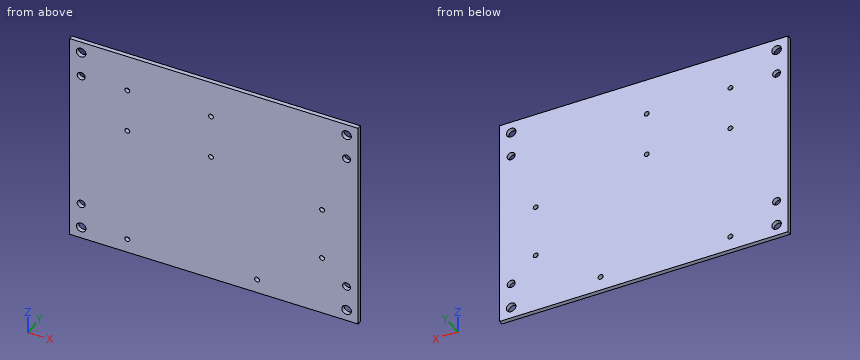
```python
from build123d import *

# Parameters (mm, degrees)
SKETCH1_W           = 200
SKETCH1_H           = 150
BOSS_EXTRUDE1_DEPTH = 3
SKETCH2_R           = 3.3
SKETCH2_R_2         = 1.7
SKETCH2_R_3         = 2.75
SKETCH2_R_4         = 1.75
CUT_EXTRUDE1_DEPTH  = 3


with BuildPart() as part:
    # Sketch1 → Boss-Extrude1 (new body)
    with BuildSketch(Plane(origin=(0, 0, 0), x_dir=(1, 0, 0), z_dir=(0, 1, 0))):
        with Locations((100, 75)):
            Rectangle(SKETCH1_W, SKETCH1_H)
    extrude(amount=BOSS_EXTRUDE1_DEPTH)

    # Sketch2 → Cut-Extrude1 (cut)
    with BuildSketch(Plane(origin=(0, 3, 0), x_dir=(1, 0, 0), z_dir=(0, 1, 0))):
        with Locations(Location((8, 142, 0), (0, 0, 270))):
            Circle(SKETCH2_R)
        with Locations(Location((8, 8, 0), (0, 0, 90))):
            Circle(SKETCH2_R)
        with Locations(Location((192, 8, 0), (0, 0, 270))):
            Circle(SKETCH2_R)
        with Locations(Location((192, 142, 0), (0, 0, 90))):
            Circle(SKETCH2_R)
        with Locations(Location((40, 57, 0), (0, 0, 270))):
            Circle(SKETCH2_R_2)
        with Locations(Location((98, 57, 0), (0, 0, 270))):
            Circle(SKETCH2_R_2)
        with Locations(Location((98, 26, 0), (0, 0, 270))):
            Circle(SKETCH2_R_2)
        with Locations(Location((40, 26, 0), (0, 0, 270))):
            Circle(SKETCH2_R_2)
        with Locations(Location((8, 124, 0), (0, 0, 270))):
            Circle(SKETCH2_R_3)
        with Locations(Location((8, 26, 0), (0, 0, 90))):
            Circle(SKETCH2_R_3)
        with Locations(Location((192, 26, 0), (0, 0, 270))):
            Circle(SKETCH2_R_3)
        with Locations(Location((192, 124, 0), (0, 0, 90))):
            Circle(SKETCH2_R_3)
        with Locations(Location((175, 108, 0), (0, 0, 270))):
            Circle(SKETCH2_R_2)
        with Locations(Location((175, 71.07, 0), (0, 0, 270))):
            Circle(SKETCH2_R_2)
        with Locations(Location((40, 140, 0), (0, 0, 270))):
            Circle(SKETCH2_R_4)
        with Locations(Location((130, 140, 0), (0, 0, 270))):
            Circle(SKETCH2_R_4)
    extrude(amount=-CUT_EXTRUDE1_DEPTH, mode=Mode.SUBTRACT)


solid = part.part
```
Here's how the part is built. I have some questions about the finished solid (model axes, mm). Round coordinates to 2 decimals unless told otherwise and drop trailing zeros. Write each loop counter-clockwise with the first axis right and the second up, starting at its lowest first coordinate (ties: lowest second). Pieces come first, ordered by that corner, then holes.
Q1. If we section it at A-A on z = -124: Write out the boundary of the cut face in (x, y).
Q2. Please list where these lines run through material, in increasing order: probe 1 along X at (y, z) = (1.5, -57); probe 2 along X at (y, z) = (1.4, -124); probe 3 along X at (y, z) = (2.2, -26).
Q3. If we section it at B-B on x = 192: Write out the boundary of the cut face in (y, z).
Q4. Will this pin go through, and if not, where does the flat tip stop? P1, Ø3, axis at x = 130, z = -140, coming from the -Y side.
Answer below:
1. outline: (0, 0) - (5.25, 0) - (5.25, 3) - (0, 3) - close; (10.75, 0) - (189.25, 0) - (189.25, 3) - (10.75, 3) - close; (194.75, 0) - (200, 0) - (200, 3) - (194.75, 3) - close
2. probe 1: x = 0 to 38.3, 41.7 to 96.3, 99.7 to 200
2. probe 2: x = 0 to 5.25, 10.75 to 189.25, 194.75 to 200
2. probe 3: x = 0 to 5.25, 10.75 to 38.3, 41.7 to 96.3, 99.7 to 189.25, 194.75 to 200
3. outline: (0, -150) - (3, -150) - (3, -145.3) - (0, -145.3) - close; (0, -138.7) - (3, -138.7) - (3, -126.75) - (0, -126.75) - close; (0, -121.25) - (3, -121.25) - (3, -28.75) - (0, -28.75) - close; (0, -23.25) - (3, -23.25) - (3, -11.3) - (0, -11.3) - close; (0, -4.7) - (3, -4.7) - (3, 0) - (0, 0) - close
4. P1: passes through
